```python
from build123d import *

# Parameters (mm, degrees)
SKETCH1_W           = 86.36
SKETCH1_H           = 101.6
SKETCH1_R           = 3.175
BOSS_EXTRUDE1_DEPTH = 6.35
CUT_EXTRUDE1_DEPTH  = 101.394283204
BOSS_EXTRUDE2_DEPTH = 86.36
SKETCH4_R           = 2.1828125
CUT_EXTRUDE2_DEPTH  = 104.736983459


with BuildPart() as part:
    # Sketch1 → Boss-Extrude1 (new body)
    with BuildSketch(Plane.XY):
        Rectangle(SKETCH1_W, SKETCH1_H)
        with Locations((-19.05, 19.05)):
            Circle(SKETCH1_R, mode=Mode.SUBTRACT)
        with Locations((19.05, 19.05)):
            Circle(SKETCH1_R, mode=Mode.SUBTRACT)
        with Locations((-19.05, -19.05)):
            Circle(SKETCH1_R, mode=Mode.SUBTRACT)
        with Locations((19.05, -19.05)):
            Circle(SKETCH1_R, mode=Mode.SUBTRACT)
    extrude(amount=BOSS_EXTRUDE1_DEPTH)

    # Sketch2 → Cut-Extrude1 (cut, through all)
    with BuildSketch(Plane(origin=(43.18, 0, 0), x_dir=(0, 0, -1), z_dir=(1, 0, 0))):
        Polygon((0, -50.8), (-6.35, -47.133825791), (-6.35, -50.8), align=None)
    extrude(amount=-CUT_EXTRUDE1_DEPTH, mode=Mode.SUBTRACT)

    # Sketch3 → Boss-Extrude2 (add, through all)
    with BuildSketch(Plane(origin=(43.18, 0, 0), x_dir=(0, 0, -1), z_dir=(1, 0, 0))):
        Polygon((0, -50.8), (9.525, -34.302216058), (0, -28.802954744), align=None)
    extrude(amount=-BOSS_EXTRUDE2_DEPTH)

    # Sketch4 → Cut-Extrude2 (cut, through all)
    with BuildSketch(Plane(origin=(0, -38.1, 21.997045256), x_dir=(-1, 0, 0), z_dir=(0, -0.8660254037844419, 0.4999999999999946))):
        with Locations(Location((31.75, 21.733825791, 0), (0, 0, 90))):
            Circle(SKETCH4_R)
        with Locations(Location((-31.75, 21.733825791, 0), (0, 0, 90))):
            Circle(SKETCH4_R)
    extrude(amount=-CUT_EXTRUDE2_DEPTH, mode=Mode.SUBTRACT)


solid = part.part
```
Can you work these out from the model? Positions are in its coordinate system, mm. A direction names the side the tool comes from. Round coordinates to 2 decimals unless told otherwise and drop trailing zeros. Order: outer loops, then holes, each group sorted by start corner. A loop starts at its lowest first (then second) coordinate and runs counter-clockwise, first axis right, second up.
(1) We'd pull the mould along Z, two halves only. Please class faces 3 (the face through (33.914, -40.691, -1.275)), 4 (the face through (-1, 3, 6.35)), 5 (the face through (16.53, 17.12, 3.13)): +Z half, -Z half, draft (parallel to the pull), parting line (faces both ways), or undercut.
Results are:
face 3: undercut
face 4: +Z half
face 5: draft
(2) If we section it at A-A (x = 19.05): Please give me the cut outline in (y, z) (3 decimals), plus the area to 3 significant figures.
Results are:
outline: (-50.8, 0) - (-34.302, -9.525) - (-28.803, 0) - (-22.225, 0) - (-22.225, 6.35) - (-47.134, 6.35) - close; (-15.875, 0) - (15.875, 0) - (15.875, 6.35) - (-15.875, 6.35) - close; (22.225, 0) - (50.8, 0) - (50.8, 6.35) - (22.225, 6.35) - close
area: 658 mm2
(3) On a 3-axis mill with a long thin cutter (end or side, diameter ignored), from which of +Z, -Z, +X, -X, +Y, -Y can I reach the whole of each face in a straight line? I mean faces 1 (the face through (-1, 12, 0)), 2 (the face through (15.88, -18.91, 3.13)). Say none if no direction works.
Results are:
face 1: -Z, +X, -X, +Y
face 2: +Z, -Z
(4) If I drill on L1, parallel to X at y = -19.5, z = 1; L2, parallel to Y at x = -19.05, z = 2 (3 decimals); L3, parallel to Y at x = -19.05, z = 4.25 (3 decimals), over which ranges is the centre line in solid material (lowest first)?
Results are:
L1: x = -43.18 to -22.19, -15.91 to 15.91, 22.19 to 43.18
L2: y = -49.645 to -22.225, -15.875 to 15.875, 22.225 to 50.8
L3: y = -48.346 to -22.225, -15.875 to 15.875, 22.225 to 50.8
(5) If we section it at D-D (z = 3.5): Count the separate pieces of the cut face and the enclosed holes in it, plus the area to 3 significant figures.
Results are:
separate pieces: 1
enclosed holes: 4
area: 8,450 mm2
(6) If we section it at C-C (x = -26.5): Please give me the cut outline in (y, z) (3 decimals), plus the area to 3 significant figures.
Results are:
outline: (-50.8, 0) - (-34.302, -9.525) - (-28.803, 0) - (50.8, 0) - (50.8, 6.35) - (-47.134, 6.35) - close
area: 738 mm2
(7) I'm going to push flat-ended pins straight in: pin 1 (5 mm diameter, centred on y = -7, z = -2, fed in from +X); pin 2 (5 mm diameter, centred on x = 34, z = -4, fed in from -Y); pin 3 (6 mm diameter, centred on x = -28.5, y = 0, fed in from -Z). Where does each tip first touch, or does it pass through?
Results are:
pin 1: stops at x = 43.18
pin 2: stops at y = -48.2
pin 3: stops at z = 0
(8) If we section it at B-B (y = -19.05): Please give me the cut outline in (x, z) (3 decimals), plus the area to 3 significant figures.
Results are:
outline: (-43.18, 0) - (-22.225, 0) - (-22.225, 6.35) - (-43.18, 6.35) - close; (-15.875, 0) - (15.875, 0) - (15.875, 6.35) - (-15.875, 6.35) - close; (22.225, 0) - (43.18, 0) - (43.18, 6.35) - (22.225, 6.35) - close
area: 468 mm2
